Can you work these out from the model? Positions are in its coordinate system, mm. Round coordinates to 2 decimals unless told otherwise and drop trailing zeros. Order: outer loops, then holes, each group sorted by start corner. A loop starts at its lowest first (then second) coordinate and runs counter-clockwise, first axis right, second up. Notation, with made-up numbers: (11, 49.25) -> (17, 49.25) arc R10 cw to (17, 64.25) -> close; hole circle Ø4 at (70.25, 61). An arc over 180 degrees is marked (long way). One line per item, written item: value.
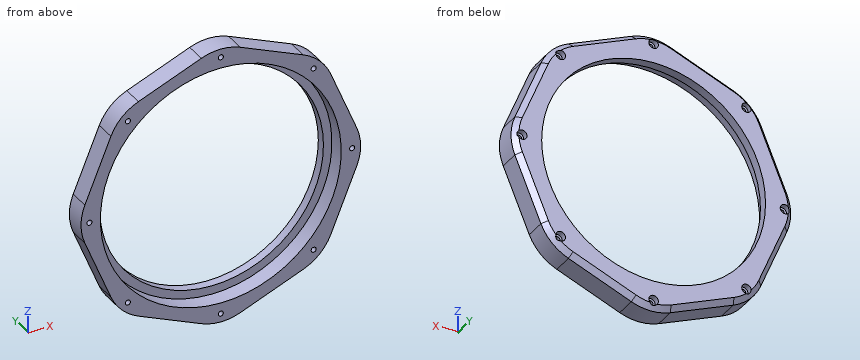
```python
from build123d import *

# Parameters (mm, degrees)
SKETCH1_R           = 66
SKETCH1_R_2         = 2.8
SKETCH1_R_3         = 1.5
BOSS_EXTRUDE1_DEPTH = 15.5
SKETCH2_R           = 71
CUT_EXTRUDE1_DEPTH  = 10
CHAMFER1_SIZE       = 3
CUT_EXTRUDE2_START  = 12
SKETCH1_6_R         = 2.8
SKETCH1_6_R_2       = 1.5
CUT_EXTRUDE2_DEPTH  = 3.5


with BuildPart() as part:
    # Sketch1 → Boss-Extrude1 (new body)
    # profile 1 of 9: a face of its own
    with BuildSketch(Plane(origin=(0, 0, 0), x_dir=(1, 0, 0), z_dir=(0, 1, 0))):
        with BuildLine():
            Line((-48.571666642, -64.807549647), (-11.480502971, -80.171212684))
            ThreePointArc((-11.480502971, -80.171212684), (0, -82.454826708), (11.480502971, -80.171212684))
            Line((11.480502971, -80.171212684), (48.571666642, -64.807549647))
            ThreePointArc((48.571666642, -64.807549647), (58.304367107, -58.304367107), (64.807549647, -48.571666642))
            Line((64.807549647, -48.571666642), (80.171212684, -11.480502971))
            ThreePointArc((80.171212684, -11.480502971), (82.454826708, 0), (80.171212684, 11.480502971))
            Line((80.171212684, 11.480502971), (64.807549647, 48.571666642))
            ThreePointArc((64.807549647, 48.571666642), (58.304367107, 58.304367107), (48.571666642, 64.807549647))
            Line((48.571666642, 64.807549647), (11.480502971, 80.171212684))
            ThreePointArc((11.480502971, 80.171212684), (0, 82.454826708), (-11.480502971, 80.171212684))
            Line((-11.480502971, 80.171212684), (-48.571666642, 64.807549647))
            ThreePointArc((-48.571666642, 64.807549647), (-58.304367107, 58.304367107), (-64.807549647, 48.571666642))
            Line((-64.807549647, 48.571666642), (-80.171212684, 11.480502971))
            ThreePointArc((-80.171212684, 11.480502971), (-82.454826708, 0), (-80.171212684, -11.480502971))
            Line((-80.171212684, -11.480502971), (-64.807549647, -48.571666642))
            ThreePointArc((-64.807549647, -48.571666642), (-58.304367107, -58.304367107), (-48.571666642, -64.807549647))
        make_face()
        with Locations(Location((0, 0, 0), (0, 0, 270))):
            Circle(SKETCH1_R, mode=Mode.SUBTRACT)
        with Locations((-77.454826708, 0)):
            Circle(SKETCH1_R_2, mode=Mode.SUBTRACT)
        with Locations((-54.768833201, -54.768833201)):
            Circle(SKETCH1_R_2, mode=Mode.SUBTRACT)
        with Locations((0, -77.454826708)):
            Circle(SKETCH1_R_2, mode=Mode.SUBTRACT)
        with Locations((54.768833201, -54.768833201)):
            Circle(SKETCH1_R_2, mode=Mode.SUBTRACT)
        with Locations((77.454826708, 0)):
            Circle(SKETCH1_R_2, mode=Mode.SUBTRACT)
        with Locations((54.768833201, 54.768833201)):
            Circle(SKETCH1_R_2, mode=Mode.SUBTRACT)
        with Locations((0, 77.454826708)):
            Circle(SKETCH1_R_2, mode=Mode.SUBTRACT)
        with Locations((-54.768833201, 54.768833201)):
            Circle(SKETCH1_R_2, mode=Mode.SUBTRACT)
    # profile 2 of 9: a face of its own
    with BuildSketch(Plane(origin=(0, 0, 0), x_dir=(1, 0, 0), z_dir=(0, 1, 0))):
        with Locations((-54.768833201, -54.768833201)):
            Circle(SKETCH1_R_2)
        with Locations(Location((-54.768833201, -54.768833201, 0), (0, 0, 270))):
            Circle(SKETCH1_R_3, mode=Mode.SUBTRACT)
    # profile 3 of 9: a face of its own
    with BuildSketch(Plane(origin=(0, 0, 0), x_dir=(1, 0, 0), z_dir=(0, 1, 0))):
        with Locations((-77.454826708, 0)):
            Circle(SKETCH1_R_2)
        with Locations(Location((-77.454826708, 0, 0), (0, 0, 270))):
            Circle(SKETCH1_R_3, mode=Mode.SUBTRACT)
    # profile 4 of 9: a face of its own
    with BuildSketch(Plane(origin=(0, 0, 0), x_dir=(1, 0, 0), z_dir=(0, 1, 0))):
        with Locations((-54.768833201, 54.768833201)):
            Circle(SKETCH1_R_2)
        with Locations(Location((-54.768833201, 54.768833201, 0), (0, 0, 270))):
            Circle(SKETCH1_R_3, mode=Mode.SUBTRACT)
    # profile 5 of 9: a face of its own
    with BuildSketch(Plane(origin=(0, 0, 0), x_dir=(1, 0, 0), z_dir=(0, 1, 0))):
        with Locations((0, 77.454826708)):
            Circle(SKETCH1_R_2)
        with Locations(Location((0, 77.454826708, 0), (0, 0, 270))):
            Circle(SKETCH1_R_3, mode=Mode.SUBTRACT)
    # profile 6 of 9: a face of its own
    with BuildSketch(Plane(origin=(0, 0, 0), x_dir=(1, 0, 0), z_dir=(0, 1, 0))):
        with Locations((54.768833201, 54.768833201)):
            Circle(SKETCH1_R_2)
        with Locations(Location((54.768833201, 54.768833201, 0), (0, 0, 270))):
            Circle(SKETCH1_R_3, mode=Mode.SUBTRACT)
    # profile 7 of 9: a face of its own
    with BuildSketch(Plane(origin=(0, 0, 0), x_dir=(1, 0, 0), z_dir=(0, 1, 0))):
        with Locations((77.454826708, 0)):
            Circle(SKETCH1_R_2)
        with Locations(Location((77.454826708, 0, 0), (0, 0, 270))):
            Circle(SKETCH1_R_3, mode=Mode.SUBTRACT)
    # profile 8 of 9: a face of its own
    with BuildSketch(Plane(origin=(0, 0, 0), x_dir=(1, 0, 0), z_dir=(0, 1, 0))):
        with Locations((54.768833201, -54.768833201)):
            Circle(SKETCH1_R_2)
        with Locations(Location((54.768833201, -54.768833201, 0), (0, 0, 270))):
            Circle(SKETCH1_R_3, mode=Mode.SUBTRACT)
    # profile 9 of 9: a face of its own
    with BuildSketch(Plane(origin=(0, 0, 0), x_dir=(1, 0, 0), z_dir=(0, 1, 0))):
        with Locations((0, -77.454826708)):
            Circle(SKETCH1_R_2)
        with Locations(Location((0, -77.454826708, 0), (0, 0, 270))):
            Circle(SKETCH1_R_3, mode=Mode.SUBTRACT)
    extrude(amount=BOSS_EXTRUDE1_DEPTH)

    # Sketch2 → Cut-Extrude1 (cut)
    with BuildSketch(Plane.XZ):
        with Locations(Location((0, 0, 0), (0, 0, 270))):
            Circle(SKETCH2_R)
    extrude(amount=-CUT_EXTRUDE1_DEPTH, mode=Mode.SUBTRACT)

    # Chamfer1
    chamfer1_edges = [part.edges().sort_by_distance(p)[0] for p in [
        (-30.026084807, 15.5, 72.489381165),
        (0, 15.5, 82.454826708),
        (30.026084807, 15.5, 72.489381165),
        (58.304367107, 15.5, 58.304367107),
        (72.489381165, 15.5, 30.026084807),
        (82.454826708, 15.5, 0),
        (72.489381165, 15.5, -30.026084807),
        (58.304367107, 15.5, -58.304367107),
        (30.026084807, 15.5, -72.489381165),
        (0, 15.5, -82.454826708),
        (-30.026084807, 15.5, -72.489381165),
        (-58.304367107, 15.5, -58.304367107),
        (-72.489381165, 15.5, -30.026084807),
        (-82.454826708, 15.5, 0),
        (-72.489381165, 15.5, 30.026084807),
        (-58.304367107, 15.5, 58.304367107),
    ]]
    chamfer(chamfer1_edges, length=CHAMFER1_SIZE)

    # Sketch1<6> → Cut-Extrude2 (cut)
    # profile 1 of 8: a face of its own
    with BuildSketch(Plane(origin=(0, 0, 0), x_dir=(1, 0, 0), z_dir=(0, 1, 0)).offset(CUT_EXTRUDE2_START)):
        with Locations(Location((-54.768833201, -54.768833201, 0), (0, 0, 270))):
            Circle(SKETCH1_6_R)
        with Locations(Location((-54.768833201, -54.768833201, 0), (0, 0, 270))):
            Circle(SKETCH1_6_R_2, mode=Mode.SUBTRACT)
    # profile 2 of 8: a face of its own
    with BuildSketch(Plane(origin=(0, 0, 0), x_dir=(1, 0, 0), z_dir=(0, 1, 0)).offset(CUT_EXTRUDE2_START)):
        with Locations(Location((0, -77.454826708, 0), (0, 0, 270))):
            Circle(SKETCH1_6_R)
        with Locations(Location((0, -77.454826708, 0), (0, 0, 270))):
            Circle(SKETCH1_6_R_2, mode=Mode.SUBTRACT)
    # profile 3 of 8: a face of its own
    with BuildSketch(Plane(origin=(0, 0, 0), x_dir=(1, 0, 0), z_dir=(0, 1, 0)).offset(CUT_EXTRUDE2_START)):
        with Locations(Location((54.768833201, -54.768833201, 0), (0, 0, 270))):
            Circle(SKETCH1_6_R)
        with Locations(Location((54.768833201, -54.768833201, 0), (0, 0, 270))):
            Circle(SKETCH1_6_R_2, mode=Mode.SUBTRACT)
    # profile 4 of 8: a face of its own
    with BuildSketch(Plane(origin=(0, 0, 0), x_dir=(1, 0, 0), z_dir=(0, 1, 0)).offset(CUT_EXTRUDE2_START)):
        with Locations(Location((77.454826708, 0, 0), (0, 0, 270))):
            Circle(SKETCH1_6_R)
        with Locations(Location((77.454826708, 0, 0), (0, 0, 270))):
            Circle(SKETCH1_6_R_2, mode=Mode.SUBTRACT)
    # profile 5 of 8: a face of its own
    with BuildSketch(Plane(origin=(0, 0, 0), x_dir=(1, 0, 0), z_dir=(0, 1, 0)).offset(CUT_EXTRUDE2_START)):
        with Locations(Location((54.768833201, 54.768833201, 0), (0, 0, 270))):
            Circle(SKETCH1_6_R)
        with Locations(Location((54.768833201, 54.768833201, 0), (0, 0, 270))):
            Circle(SKETCH1_6_R_2, mode=Mode.SUBTRACT)
    # profile 6 of 8: a face of its own
    with BuildSketch(Plane(origin=(0, 0, 0), x_dir=(1, 0, 0), z_dir=(0, 1, 0)).offset(CUT_EXTRUDE2_START)):
        with Locations(Location((0, 77.454826708, 0), (0, 0, 270))):
            Circle(SKETCH1_6_R)
        with Locations(Location((0, 77.454826708, 0), (0, 0, 270))):
            Circle(SKETCH1_6_R_2, mode=Mode.SUBTRACT)
    # profile 7 of 8: a face of its own
    with BuildSketch(Plane(origin=(0, 0, 0), x_dir=(1, 0, 0), z_dir=(0, 1, 0)).offset(CUT_EXTRUDE2_START)):
        with Locations(Location((-54.768833201, 54.768833201, 0), (0, 0, 270))):
            Circle(SKETCH1_6_R)
        with Locations(Location((-54.768833201, 54.768833201, 0), (0, 0, 270))):
            Circle(SKETCH1_6_R_2, mode=Mode.SUBTRACT)
    # profile 8 of 8: a face of its own
    with BuildSketch(Plane(origin=(0, 0, 0), x_dir=(1, 0, 0), z_dir=(0, 1, 0)).offset(CUT_EXTRUDE2_START)):
        with Locations(Location((-77.454826708, 0, 0), (0, 0, 270))):
            Circle(SKETCH1_6_R)
        with Locations(Location((-77.454826708, 0, 0), (0, 0, 270))):
            Circle(SKETCH1_6_R_2, mode=Mode.SUBTRACT)
    extrude(amount=CUT_EXTRUDE2_DEPTH, mode=Mode.SUBTRACT)


solid = part.part
```
Q1. Will these pins go through, and if not, where does the flat tip stop? pin 1 Ø4 at (x, z) = (54.77, 54.77) entering from +Y; pin 2 Ø3 at (x, y) = (-60.5, 5) entering from -Z; pin 3 Ø6 at (y, z) = (3, 28) entering from -X.
Answers below:
pin 1: y = 12
pin 2: z = -57.59
pin 3: x = -74.57
Q2. I want a section at C-C on y = 7.75. Give the number of separate pieces and of enclosed holes in the cut face, plus the area to 3 significant figures.
Answers below:
separate pieces: 1
enclosed holes: 9
area: 4,350 mm^2
Q3. I want a section at B-B on x = 23. List the corners of the cut face in (y, z) for me, plus the area to 3 significant figures.
Answers below:
outline: (0, -75.4) -> (12.5, -75.4) -> (15.5, -72.15) -> (15.5, -61.86) -> (10, -61.86) -> (10, -67.17) -> (0, -67.17) -> close; (0, 67.17) -> (10, 67.17) -> (10, 61.86) -> (15.5, 61.86) -> (15.5, 72.15) -> (12.5, 75.4) -> (0, 75.4) -> close
area: 304 mm^2
Q4. Please list where these lines run through material, in increasing order: line 1 along X through (y, z) = (8.5, 0); line 2 along Z through (x, y) = (55.5, 12.5); line 3 along X through (y, z) = (2, -38.5).
Answers below:
line 1: -82.45 to -78.95, -75.95 to -71, 71 to 75.95, 78.95 to 82.45
line 2: -60.78 to -57.47, -52.07 to -35.72, 35.72 to 52.07, 57.47 to 60.78
line 3: -68.98 to -59.66, 59.66 to 68.98
Q5. I want a section at A-A on z = -31. List the corners of the cut face in (x, y) for me.
Answers below:
outline: (-72.09, 0) -> (-63.87, 0) -> (-63.87, 10) -> (-58.27, 10) -> (-58.27, 15.5) -> (-68.84, 15.5) -> (-72.09, 12.5) -> close; (58.27, 10) -> (63.87, 10) -> (63.87, 0) -> (72.09, 0) -> (72.09, 12.5) -> (68.84, 15.5) -> (58.27, 15.5) -> close
